Geometry check sheet. Reference: the model listing, model coordinates, mm. Face numbers are marked on the shaded views. A direction names the side the tool comes from. Round coordinates to 2 decimals unless told otherwise and drop trailing zeros. Write each loop counter-clockwise with the first axis right and the second up, starting at its lowest first coordinate (ties: lowest second). Pieces come first, ordered by that corner, then holes. Notation, with made-up numbers: M 58,48.5 L 92,48.5 A13 cw 92,71.5 Z; hole C 18,78.5 d11. An arc over 180 degrees is marked long. Use a Markdown table: item, result.
```python
from build123d import *

# Parameters (mm, degrees)
SKETCH1_R           = 2.5
BOSS_EXTRUDE1_DEPTH = 3
SKETCH2_R           = 2.5
BOSS_EXTRUDE2_DEPTH = 5
SKETCH4_R           = 1.05
CUT_EXTRUDE2_DEPTH  = 4.5
SKETCH6_W           = 90
SKETCH6_H           = 60
SKETCH6_W_2         = 82
SKETCH6_H_2         = 52
BOSS_EXTRUDE3_DEPTH = 22
SKETCH7_W           = 13.75
SKETCH7_H           = 12
CUT_EXTRUDE3_DEPTH  = 20
SKETCH8_R           = 1.5
CUT_EXTRUDE4_DEPTH  = 10
SKETCH10_W          = 6.5
SKETCH10_H          = 5.005531991
CUT_EXTRUDE5_DEPTH  = 10


with BuildPart() as part:
    # Sketch1 → Boss-Extrude1 (new body)
    with BuildSketch(Plane(origin=(0, 0, 0), x_dir=(1, 0, 0), z_dir=(0, 1, 0))):
        with BuildLine():
            Line((-45, 30), (-10, 30))
            ThreePointArc((-10, 30), (0, 40), (10, 30))
            Line((10, 30), (45, 30))
            Line((45, 30), (45, -30))
            Line((45, -30), (10, -30))
            ThreePointArc((10, -30), (0, -40), (-10, -30))
            Line((-10, -30), (-45, -30))
            Line((-45, -30), (-45, 30))
        make_face()
        with Locations((0, 34)):
            Circle(SKETCH1_R, mode=Mode.SUBTRACT)
        with Locations((0, -34)):
            Circle(SKETCH1_R, mode=Mode.SUBTRACT)
    extrude(amount=BOSS_EXTRUDE1_DEPTH)

    # Sketch2 → Boss-Extrude2 (add)
    with BuildSketch(Plane(origin=(0, 3, 0), x_dir=(1, 0, 0), z_dir=(0, 1, 0))):
        with Locations((-35.17920076, 22.499548704)):
            Circle(SKETCH2_R)
        with Locations((31, 22.499548704)):
            Circle(SKETCH2_R)
        with Locations((31, -3.500451296)):
            Circle(SKETCH2_R)
        with Locations((-35.17920076, -3.500451296)):
            Circle(SKETCH2_R)
        with Locations((-35.220554781, -9.500308782)):
            Circle(SKETCH2_R)
        with Locations((31, -9.500308782)):
            Circle(SKETCH2_R)
        with Locations((-35.310155161, -22.5)):
            Circle(SKETCH2_R)
        with Locations((31, -22.5)):
            Circle(SKETCH2_R)
    extrude(amount=BOSS_EXTRUDE2_DEPTH)

    # Sketch4 → Cut-Extrude2 (cut)
    with BuildSketch(Plane(origin=(0, 8, 0), x_dir=(1, 0, 0), z_dir=(0, 1, 0))):
        with Locations((-35.17920076, 22.499548704)):
            Circle(SKETCH4_R)
        with Locations((31, 22.499548704)):
            Circle(SKETCH4_R)
        with Locations((31, -3.500451296)):
            Circle(SKETCH4_R)
        with Locations((31, -9.500308782)):
            Circle(SKETCH4_R)
        with Locations((-35.17920076, -3.500451296)):
            Circle(SKETCH4_R)
        with Locations((-35.220554781, -9.500308782)):
            Circle(SKETCH4_R)
        with Locations((-35.310155161, -22.5)):
            Circle(SKETCH4_R)
        with Locations((31, -22.5)):
            Circle(SKETCH4_R)
    extrude(amount=-CUT_EXTRUDE2_DEPTH, mode=Mode.SUBTRACT)

    # Sketch6 → Boss-Extrude3 (add)
    with BuildSketch(Plane(origin=(0, 3, 0), x_dir=(1, 0, 0), z_dir=(0, 1, 0))):
        Rectangle(SKETCH6_W, SKETCH6_H)
        Rectangle(SKETCH6_W_2, SKETCH6_H_2, mode=Mode.SUBTRACT)
    extrude(amount=BOSS_EXTRUDE3_DEPTH)

    # Sketch7 → Cut-Extrude3 (cut)
    with BuildSketch(Plane.ZY.offset(-41)):
        with Locations((-11.125, 9)):
            Rectangle(SKETCH7_W, SKETCH7_H)
    extrude(amount=-CUT_EXTRUDE3_DEPTH, mode=Mode.SUBTRACT)

    # Sketch8 → Cut-Extrude4 (cut)
    with BuildSketch(Plane(origin=(0, 25, 0), x_dir=(1, 0, 0), z_dir=(0, 1, 0))):
        with Locations((-42.5, 27.5)):
            Circle(SKETCH8_R)
        with Locations((42.5, 27.5)):
            Circle(SKETCH8_R)
        with Locations((-42.5, -28)):
            Circle(SKETCH8_R)
        with Locations((42.5, -27.5)):
            Circle(SKETCH8_R)
    extrude(amount=-CUT_EXTRUDE4_DEPTH, mode=Mode.SUBTRACT)

    # Sketch10 → Cut-Extrude5 (cut)
    with BuildSketch(Plane(origin=(-41, 0, 0), x_dir=(0, 0, -1), z_dir=(1, 0, 0))):
        with Locations((-16.050308782, 5.502765995)):
            Rectangle(SKETCH10_W, SKETCH10_H)
    extrude(amount=-CUT_EXTRUDE5_DEPTH, mode=Mode.SUBTRACT)


solid = part.part
```
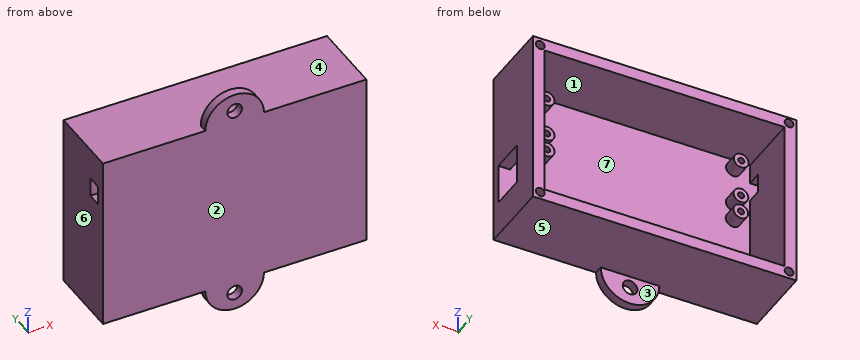
Item 1: Cross-section at D-D, the plane y = 7. Count the separate pieces of the cut face and the enclosed holes in it, and give its area (3 significant figures).
Outcome:
| item | result |
|---|---|
| separate pieces | 10 |
| enclosed holes | 8 |
| area | 1,180 mm2 |
Item 2: Material ranges on line 1 along Z through (x, y) = (-42.5, 17.5); line 2 along Z through (x, y) = (0, 2.3); line 3 along Z through (x, y) = (21.5, 19.25), recorded low to high. Write a range as from..to.
Outcome:
| item | result |
|---|---|
| line 1 | z = -30..-29, -26..26.5, 29.5..30 |
| line 2 | z = -40..-36.5, -31.5..31.5, 36.5..40 |
| line 3 | z = -30..-26, 26..30 |
Item 3: Mould release check, pull along Z, two halves, no side actions. Record for the marked faces 4, 5, 6 and 7: +Z half, -Z half, draft (parallel to the pull), parting line (faces both ways), or undercut.
Outcome:
| item | result |
|---|---|
| face 4 | +Z half |
| face 5 | -Z half |
| face 6 | draft |
| face 7 | undercut |
Item 4: Go/stop test with flat-tipped pins: pin 1 (4.5 mm diameter, centred on x = -44, y = 6.5, fed in from -Z); pin 2 (2.5 mm diameter, centred on x = 42.5, z = 27.5, fed in from -Y); pin 3 (0.9 mm diameter, centred on x = -43, z = 28.5, fed in from +Y); pin 4 (2.5 mm diameter, centred on x = -35.5, z = 9.5, fed in from +Y). Record where each tip stops, or that it passes through.
Outcome:
| item | result |
|---|---|
| pin 1 | stops at z = -30 |
| pin 2 | stops at y = 0 |
| pin 3 | stops at y = 15 |
| pin 4 | stops at y = 8 |
Item 5: Access from +Z, -Z, +X, -X, +Y, -Y to the whole of each face (thin tool, end or side, straight path). Record for the marked faces 1, 2 and 3.
Outcome:
| item | result |
|---|---|
| face 1 | +Y |
| face 2 | +Z, -Z, +X, -X, -Y |
| face 3 | -Z, +X, -X, +Y |
Item 6: Cross-section at C-C, the plane x = 42.5. Record the cut outline in (y, z), and give its area (4 significant figures).
Outcome:
| item | result |
|---|---|
| outline | M 0,-30 L 25,-30 L 25,-29 L 15,-29 L 15,-26 L 25,-26 L 25,26 L 15,26 L 15,29 L 25,29 L 25,30 L 0,30 Z; hole M 3,-18 L 15,-18 L 15,-4.25 L 3,-4.25 Z |
| area | 1,275 mm2 |
Item 7: Cross-section at A-A, the plane z = -14.5. Record the cut outline in (x, y), and give its area (3 significant figures).
Outcome:
| item | result |
|---|---|
| outline | M -45,0 L 45,0 L 45,3 L -41,3 L -41,25 L -45,25 Z; M 41,15 L 45,15 L 45,25 L 41,25 Z |
| area | 398 mm2 |
Item 8: Cross-section at B-B, the plane y = 22.5. Record the cut outline in (x, z).
Outcome:
| item | result |
|---|---|
| outline | M -45,-30 L 45,-30 L 45,30 L -45,30 Z; hole C -42.5,-27.5 d3; hole C -42.5,28 d3; hole M -41,-26 L 41,-26 L 41,26 L -41,26 Z; hole C 42.5,-27.5 d3; hole C 42.5,27.5 d3 |
